Autodesk Inventor part; units mm, degrees
ref_plane "Startebene" through (0, 0, 0) normal (0, 0, 1) x (1, 0, 0)
ref_plane "Endebene" through (0, 0, 320) normal (0, 0, 1) x (1, 0, 0)
ref_plane "Startebene1" through (0, 0, 0) normal (0, 0, 1) x (1, 0, 0)
ref_plane "Startebene" through (0, 0, 0) normal (0, 0, 1) x (1, 0, 0)
ref_plane "Endebene" through (0, 0, 320) normal (0, 0, 1) x (1, 0, 0)
ref_plane "Startebene1" through (0, 0, 0) normal (0, 0, 1) x (1, 0, 0)
ref_plane "Endebene1" through (0, 0, 60) normal (0, 0, 1) x (1, 0, 0)
ref_plane "Startebene2" through (0, 0, 10) normal (0, 0, 1) x (1, 0, 0)
ref_plane "Endebene2" through (0, 0, 50) normal (0, 0, 1) x (1, 0, 0)
sketch "Skizze" plane through (0, 0, 0) normal (0, 0, 1) x (1, 0, 0)
  line L0 (-10, 9) -> (-10, 3.3)
  arc A0 (-10, 3.3) -> (-9.7, 3) centre (-9.7, 3.3) ccw
  line L1 (-9.7, 3) -> (-8, 3)
  line L2 (-8, 3) -> (-8, 6)
  line L3 (-8, 6) -> (-7.0607, 6)
  line L4 (-7.0607, 6) -> (-4, 2.9393)
  line L5 (-4, 2.9393) -> (-4, 0.3)
  line L6 (-4, 0.3) -> (-3.7, 0)
  line L7 (-3.7, 0) -> (-4, -0.3)
  line L8 (-4, -0.3) -> (-4, -2.9393)
  line L9 (-4, -2.9393) -> (-7.0607, -6)
  line L10 (-7.0607, -6) -> (-8, -6)
  line L11 (-8, -6) -> (-8, -3)
  line L12 (-8, -3) -> (-9.7, -3)
  arc A1 (-9.7, -3) -> (-10, -3.3) centre (-9.7, -3.3) ccw
  line L13 (-10, -3.3) -> (-10, -9)
  arc A2 (-10, -9) -> (-9, -10) centre (-9, -9) ccw
  line L14 (-9, -10) -> (-3.3, -10)
  arc A3 (-3.3, -10) -> (-3, -9.7) centre (-3.3, -9.7) ccw
  line L15 (-3, -9.7) -> (-3, -8)
  line L16 (-3, -8) -> (-6, -8)
  line L17 (-6, -8) -> (-6, -7.0607)
  line L18 (-6, -7.0607) -> (-2.9393, -4)
  line L19 (-2.9393, -4) -> (-0.3, -4)
  line L20 (-0.3, -4) -> (0, -3.7)
  line L21 (0, -3.7) -> (0.3, -4)
  line L22 (0.3, -4) -> (2.9393, -4)
  line L23 (2.9393, -4) -> (6, -7.0607)
  line L24 (6, -7.0607) -> (6, -8)
  line L25 (6, -8) -> (3, -8)
  line L26 (3, -8) -> (3, -9.7)
  arc A4 (3, -9.7) -> (3.3, -10) centre (3.3, -9.7) ccw
  line L27 (3.3, -10) -> (9, -10)
  arc A5 (9, -10) -> (10, -9) centre (9, -9) ccw
  line L28 (10, -9) -> (10, -3.3)
  arc A6 (10, -3.3) -> (9.7, -3) centre (9.7, -3.3) ccw
  line L29 (9.7, -3) -> (8, -3)
  line L30 (8, -3) -> (8, -6)
  line L31 (8, -6) -> (7.0607, -6)
  line L32 (7.0607, -6) -> (4, -2.9393)
  line L33 (4, -2.9393) -> (4, -0.3)
  line L34 (4, -0.3) -> (3.7, 0)
  line L35 (3.7, 0) -> (4, 0.3)
  line L36 (4, 0.3) -> (4, 2.9393)
  line L37 (4, 2.9393) -> (7.0607, 6)
  line L38 (7.0607, 6) -> (8, 6)
  line L39 (8, 6) -> (8, 3)
  line L40 (8, 3) -> (9.7, 3)
  arc A7 (9.7, 3) -> (10, 3.3) centre (9.7, 3.3) ccw
  line L41 (10, 3.3) -> (10, 9)
  arc A8 (10, 9) -> (9, 10) centre (9, 9) ccw
  line L42 (9, 10) -> (3.3, 10)
  arc A9 (3.3, 10) -> (3, 9.7) centre (3.3, 9.7) ccw
  line L43 (3, 9.7) -> (3, 8)
  line L44 (3, 8) -> (6, 8)
  line L45 (6, 8) -> (6, 7.0607)
  line L46 (6, 7.0607) -> (2.9393, 4)
  line L47 (2.9393, 4) -> (0.3, 4)
  line L48 (0.3, 4) -> (0, 3.7)
  line L49 (0, 3.7) -> (-0.3, 4)
  line L50 (-0.3, 4) -> (-2.9393, 4)
  line L51 (-2.9393, 4) -> (-6, 7.0607)
  line L52 (-6, 7.0607) -> (-6, 8)
  line L53 (-6, 8) -> (-3, 8)
  line L54 (-3, 8) -> (-3, 9.7)
  arc A10 (-3, 9.7) -> (-3.3, 10) centre (-3.3, 9.7) ccw
  line L55 (-3.3, 10) -> (-9, 10)
  arc A11 (-9, 10) -> (-10, 9) centre (-9, 9) ccw
  circle A12 centre (0, 0) radius 2.75
  dimension "d2" = 5.5
  dimension "d3" = 10
  dimension "d4" = 10
  dimension "d5" = 5.7
  dimension "d6" = 5.7
  dimension "d7" = 1.7
  dimension "d8" = 3
  dimension "d9" = 0.3
  dimension "d10" = 90
  dimension "d11" = 45
  dimension "d12" = 45
  dimension "d13" = 45
  dimension "d14" = 90
  dimension "d15" = 90
  dimension "d16" = 45
  dimension "d17" = 45
  dimension "d18" = 45
  dimension "d19" = 45
  dimension "d20" = 90
  dimension "d21" = 90
  dimension "d22" = 45
  dimension "d23" = 45
  dimension "d24" = 90
  dimension "d25" = 90
  dimension "d26" = 90
  dimension "d27" = 90
  dimension "d28" = 90
  dimension "d29" = 90
  dimension "d30" = 90
  dimension "d31" = 90
  dimension "d32" = 90
  dimension "d33" = 90
  dimension "d34" = 90
  dimension "d35" = 90
  dimension "d36" = 90
  dimension "d37" = 90
  dimension "d38" = 90
  dimension "d39" = 4
  dimension "d40" = 6
  dimension "d41" = 13
  dimension "d42" = 14
  dimension "d43" = 16
  dimension "d44" = 18
  dimension "d45" = 3
  dimension "d46" = 9
  dimension "d47" = 7
  dimension "d48" = 1
  dimension "d49" = 7
  dimension "d50" = 1.5
  dimension "d51" = 1.8663
  dimension "d52" = 3.3663
  dimension "d53" = 1.5
  dimension "d54" = 1.8663
  dimension "d55" = 3.3663
  dimension "d56" = 4
  dimension "d57" = 10.8187
  dimension "d58" = 1.9092
  dimension "d59" = 5
  dimension "d60" = 13
  dimension "d61" = 13
  dimension "d62" = 16.0513
  dimension "d63" = 3.3234
  dimension "d64" = 14
  dimension "d65" = 12.685
extrude "Körper" add sketch "Skizze" along normal up to surface (40 mm away) from surface at 10
sketch "Skizze13" plane through (0, 0, 0) normal (0, 0, 1) x (1, 0, 0)
  line L0 (0, 0) -> (10, 0)
ref_plane "Arbeitsebene12" through (0, 0, 0) normal (0, -1, 0) x (1, 0, 0)
sketch "Skizze14" plane through (0, 0, 0) normal (0, -1, 0) x (1, 0, 0)
  line L0 (-2, 10) -> (12, 10)
  line L1 (-2, 50) -> (12, 50)
  dimension "d80" = 40
ref_plane "Arbeitsebene13" through (-9, 0, 10) normal (0, 0, -1) x (-1, 0, 0)
split "Trennen1" plane through (-9, 0, 10) removes the side toward (0, 0, -1)
ref_plane "Arbeitsebene14" through (-9, 50, 50) normal (0, 0, 1) x (1, 0, 0)
split "Trennen2" plane through (-9, 50, 50) removes the side toward (0, 0, 1)
equation "\"G_OFFSET_START\" = 0"
equation "\"G_OFFSET_END\" = 0"
equation "\"G_L\" = d80"
equation "\"G_OFFSET_START1\" = 0"
equation "\"G_OFFSET_END1\" = 0"
properties part number "Alu Profil 20x20 - AP2020" material "Aluminium 6061"
Geometry check sheet. Reference: the model listing, model coordinates, mm. A direction names the side the tool comes from. Coordinates: 2 decimals unless noted, no trailing zeros. Order: outer loops, then holes, each group sorted by start corner. A loop starts at its lowest first (then second) coordinate and runs counter-clockwise, first axis right, second up. Notation, with made-up numbers: (65, 6.25) - (102, 6.25) arc R18 ccw to (102, 34.25) - close; hole circle Ø10 at (52.5, 18.25). An arc over 180 degrees is marked (long way). Answer as a JSON object with one key per item and string values. Group by question number.
Item 1: Depth check by flat-ended pin: pin 1 Ø0.8 at (y, z) = (-2.5, 23.5) entering from +X; pin 2 Ø6 at (x, z) = (-2.5, 41.5) entering from -Y; pin 3 Ø1.3 at (x, z) = (2, 34) entering from -Y; pin 4 Ø1.3 at (x, z) = (1.5, 38) entering from +Y. Enter the tip coordinate at first touch or a pass-through.
Item 2: Draft check along Y on faces 4 (the face through (-10, -6, 30)), 5 (the face through (-8, 4, 30)), 6 (the face through (6, 10, 30)), 7 (the face through (-2, -4, 30)). Enter one of: +Y half, -Y half, draft (parallel to the pull), parting line (faces both ways), or undercut.
Item 3: Sectioned sample at B-B, the plane x = 5.5. Record the cut outline in (y, z), and give its area (3 significant figures).
Item 4: Sectioned sample at C-C, the plane y = 0.75. Record the cut outline in (x, z).
Item 5: Sectioned sample at A-A, the plane y = 8.5. Record the cut outline in (x, z).
Item 6: Tool access check on faces 1 (the face through (3, 9, 30)), 2 (the face through (-4, -2, 30)), 3 (the face through (-4.49, -5.55, 29.72)). Record the directions out of +Z, -Z, +X, -X, +Y, -Y that give a thin tool (end or side, any length) a straight path to the whole face; none if there is none.
Item 7: Scan lines: probe 1 along Y at (x, z) = (8.5, 27.5); probe 2 along Y at (x, z) = (5.75, 41); probe 3 along Y at (x, z) = (7.5, 45). Record each from-to range of solid material in increasing order.
Resolved:
{
 "1": {"pin 1": "x = 4", "pin 2": "y = -10", "pin 3": "y = -4", "pin 4": "y = 4"},
 "2": {"face 4": "draft", "face 5": "undercut", "face 6": "+Y half", "face 7": "-Y half"},
 "3": {"outline": "(-10, 10) - (-8, 10) - (-8, 50) - (-10, 50) - close; (-6.56, 10) - (-4.44, 10) - (-4.44, 50) - (-6.56, 50) - close; (4.44, 10) - (6.56, 10) - (6.56, 50) - (4.44, 50) - close; (8, 10) - (10, 10) - (10, 50) - (8, 50) - close", "area": "330 mm^2"},
 "4": {"outline": "(-4, 10) - (-2.65, 10) - (-2.65, 50) - (-4, 50) - close; (2.65, 10) - (4, 10) - (4, 50) - (2.65, 50) - close"},
 "5": {"outline": "(-10, 10) - (-3, 10) - (-3, 50) - (-10, 50) - close; (3, 10) - (10, 10) - (10, 50) - (3, 50) - close"},
 "6": {"face 1": "+Z, -Z, +Y", "face 2": "+Z, -Z, -X", "face 3": "+Z, -Z"},
 "7": {"probe 1": "-10 to -3, 3 to 10", "probe 2": "-10 to -8, -6.81 to -4.69, 4.69 to 6.81, 8 to 10", "probe 3": "-10 to -6, 6 to 10"}
}
